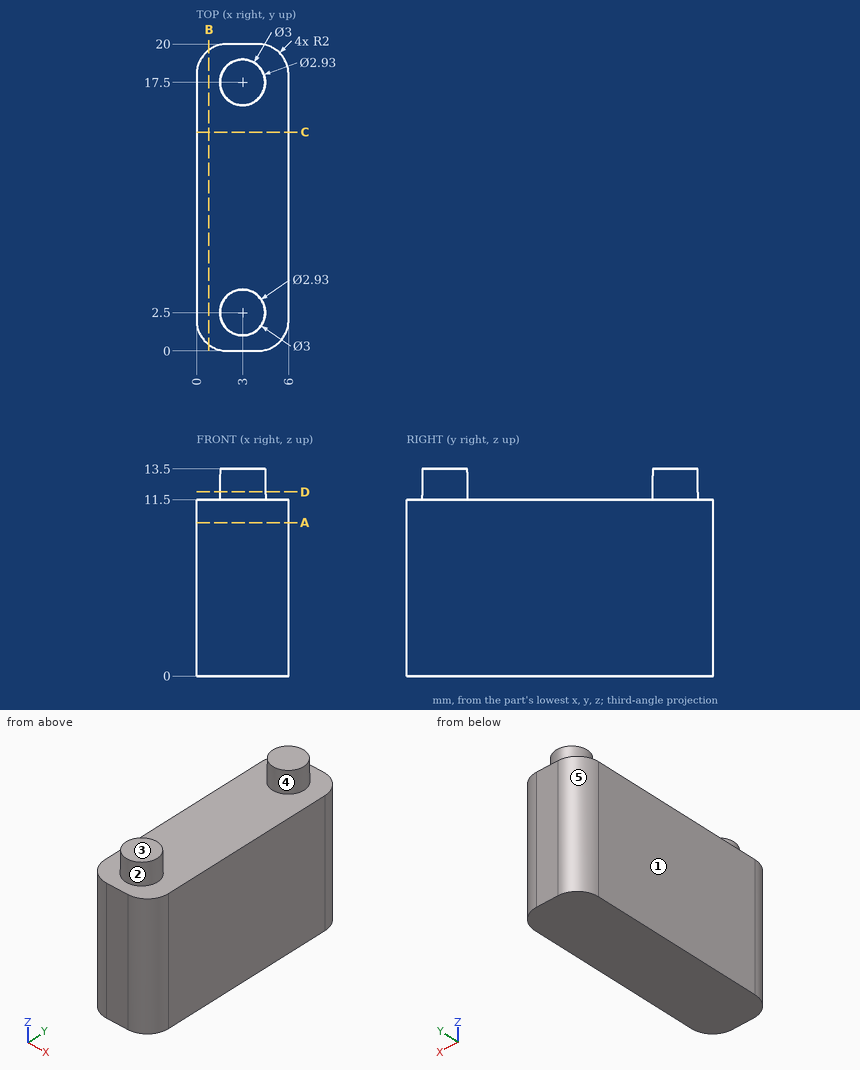
Geometry: see drawing. Coordinates: mm, zero at the bounding-box minimum. A direction names the side the tool comes from. Coordinates: 2 decimals unless noted, no trailing zeros. Write each loop counter-clockwise with the first axis right and the second up, starting at its lowest first coordinate (ties: lowest second). Pieces come first, ordered by that corner, then holes. Notation, with made-up numbers: M 26.5,-22.5 L 47.5,-22.5 A22 ccw 47.5,15.5 Z; hole C 51,-0.5 d6. An arc over 180 degrees is marked long. Use CSV: the item, a comma, the result in double quotes. Start each with the question number.
1. First-contact query: P1, Ø1.8, axis at x = 4, y = 14, coming from the +Z side. Flat tip, straight axial feed; report the tip coordinate or a pass-through.
2. Reachability of the marked faces 1 and 2 from +Z, -Z, +X, -X, +Y, -Y: full face, straight path, thin tool, end or side. Return the list, or none.
3. Cut plane A-A on z = 10. Return the cut outline in (x, y), plus the area to 3 significant figures.
4. Cut plane D-D on z = 12. Return the cut outline in (x, y), plus the area to 3 significant figures.
5. Mould query, pull axis Y, two halves, no side actions, for the marked faces 3, 4 and 5. Classes: pulls with the +Y half, pulls with the -Y half, needs draft (parallel to the pull), parting line crosses it, or undercut.
6. Ray query, probe 1 along Z at (x, y) = (1, 6.75); probe 2 along X at (y, z) = (18.5, 2.75); probe 3 along Y at (x, z) = (4.4, 10.25). Return the intervals inside material, ascending.
7. Cut plane B-B on x = 0.8. Return the cut outline in (y, z), plus the area to 3 significant figures.
8. Cut plane C-C on y = 14.25. Return the cut outline in (x, z), plus the area to 3 significant figures.
Entries:
1,P1,"z = 11.5"
2,face 1,"+Z, -Z, -X, +Y, -Y"
2,face 2,"+Z"
3,outline,"M 0,2 A2 ccw 2,0 L 4,0 A2 ccw 6,2 L 6,18 A2 ccw 4,20 L 2,20 A2 ccw 0,18 Z"
3,area,"117 mm²"
4,outline,"C 3,2.5 d2.98; C 3,17.5 d2.98"
4,area,"14.0 mm²"
5,face 3,"needs draft"
5,face 4,"undercut"
5,face 5,"pulls with the +Y half"
6,probe 1,"0 to 11.5"
6,probe 2,"0.06 to 5.94"
6,probe 3,"0.04 to 19.96"
7,outline,"M 0.4,0 L 19.6,0 L 19.6,11.5 L 0.4,11.5 Z"
7,area,"221 mm²"
8,outline,"M 0,0 L 6,0 L 6,11.5 L 0,11.5 Z"
8,area,"69.0 mm²"
